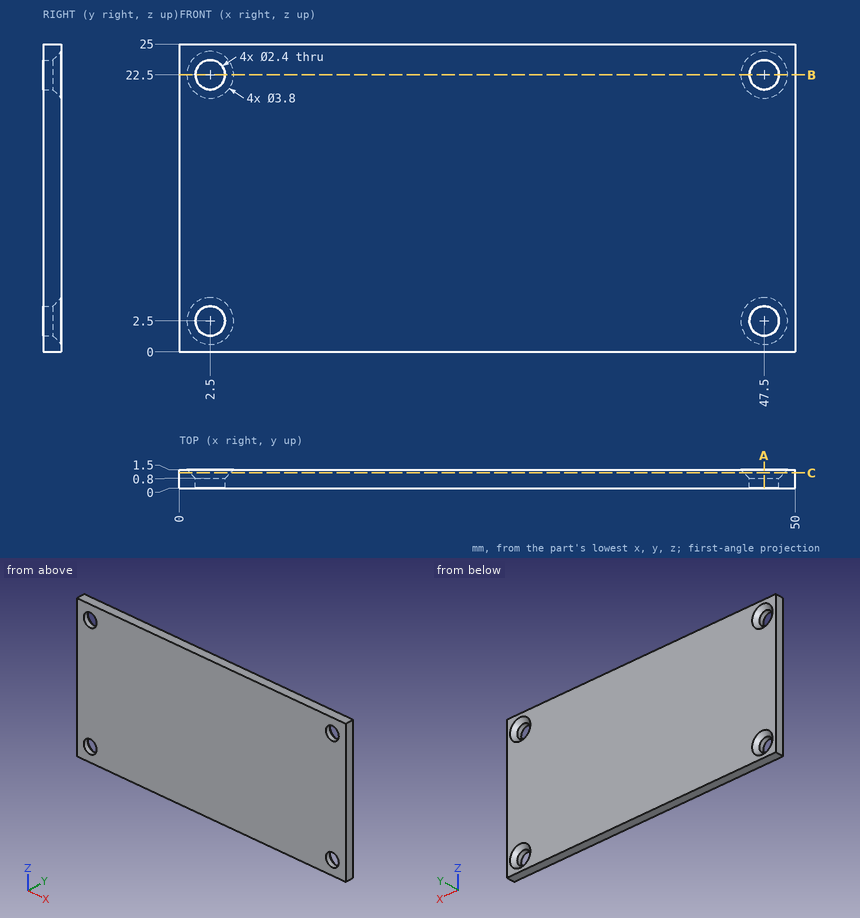
Could you check a few things on this drawing? It's one solid part, dimensions in mm from its lowest x, y, z. Give positions to 0.01 mm unless a question says otherwise; leave off trailing zeros. Order: outer loops, then holes, each group sorted by start corner. A loop starts at its lowest first (then second) coordinate and runs counter-clockwise, first axis right, second up. Notation, with made-up numbers: (78, 40.5) -> (123, 40.5) arc R16 cw to (123, 46.5) -> close; hole circle Ø11 at (47.5, 88). An arc over 180 degrees is marked (long way). Answer in a Markdown table with one row per item. Add a question column.
Item 1: Imagine slicing it at A-A (x = 47.5). List the corners of the cut face in (y, z) for me.
Item 2: Imagine slicing it at C-C (y = 1.25). List the corners of the cut face in (x, z) for me.
Item 3: I'm going to push a flat-ended pin straight in: P1, Ø3, axis at x = 47.5, z = 2.5, coming from the +Y side. Where does the tip first touch, or does it pass through?
Item 4: Please list where these lines run through material, in increasing order: probe 1 along X at (y, z) = (0.65, 2.5); probe 2 along Z at (x, y) = (2.5, 0.55).
Item 5: Imagine slicing it at B-B (z = 22.5). List the corners of the cut face in (x, y) for me, and give its area (3 significant figures).
Result:
| question | item | result |
|---|---|---|
| 1 | outline | (0, 0) -> (1.5, 0) -> (1.5, 0.6) -> (0.8, 1.3) -> (0, 1.3) -> close; (0, 3.7) -> (0.8, 3.7) -> (1.5, 4.4) -> (1.5, 20.6) -> (0.8, 21.3) -> (0, 21.3) -> close; (0, 23.7) -> (0.8, 23.7) -> (1.5, 24.4) -> (1.5, 25) -> (0, 25) -> close |
| 2 | outline | (0, 0) -> (50, 0) -> (50, 25) -> (0, 25) -> close; hole circle Ø3.3 at (2.5, 2.5); hole circle Ø3.3 at (2.5, 22.5); hole circle Ø3.3 at (47.5, 2.5); hole circle Ø3.3 at (47.5, 22.5) |
| 3 | P1 | y = 1.1 |
| 4 | probe 1 | 0 to 1.3, 3.7 to 46.3, 48.7 to 50 |
| 4 | probe 2 | 0 to 1.3, 3.7 to 21.3, 23.7 to 25 |
| 5 | outline | (0, 0) -> (1.3, 0) -> (1.3, 0.8) -> (0.6, 1.5) -> (0, 1.5) -> close; (3.7, 0) -> (46.3, 0) -> (46.3, 0.8) -> (45.6, 1.5) -> (4.4, 1.5) -> (3.7, 0.8) -> close; (48.7, 0) -> (50, 0) -> (50, 1.5) -> (49.4, 1.5) -> (48.7, 0.8) -> close |
| 5 | area | 66.8 mm2 |
